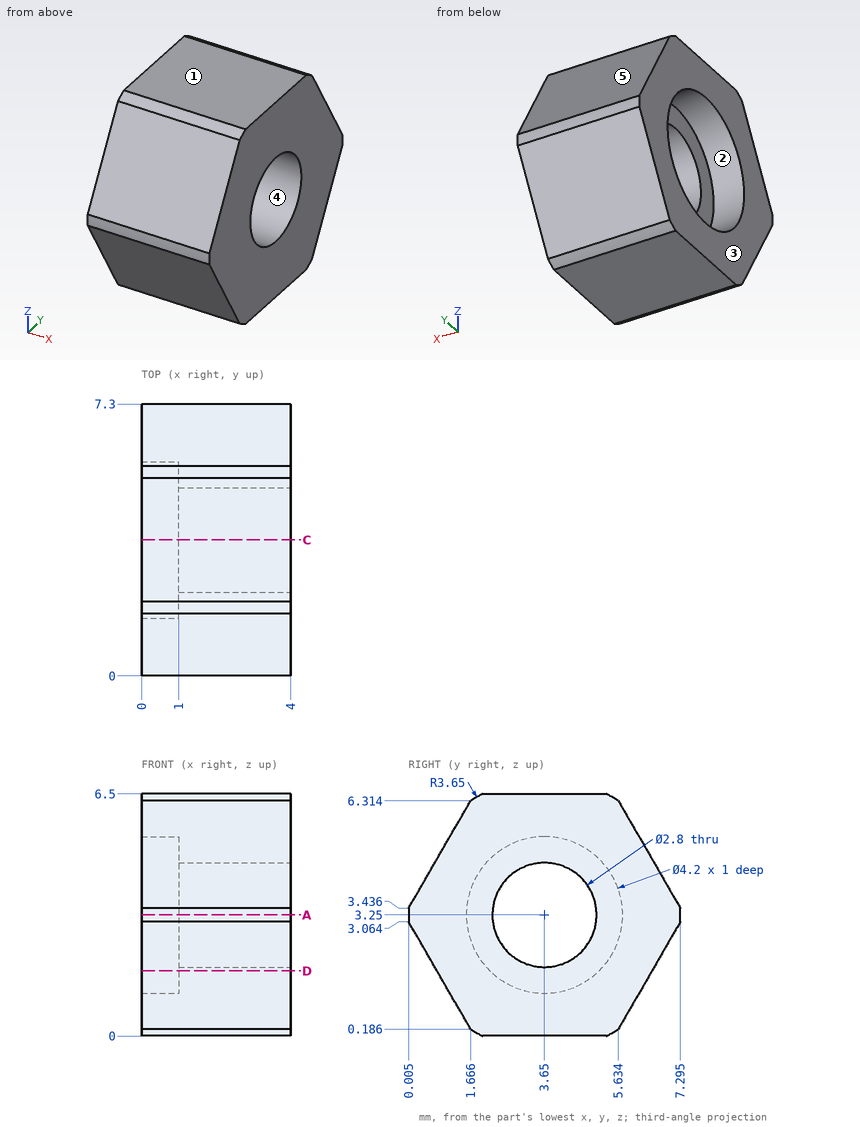
Geometry: see drawing. Coordinates: mm, zero at the bounding-box minimum. A direction names the side the tool comes from. Coordinates: 2 decimals unless noted, no trailing zeros. Order: outer loops, then holes, each group sorted by start corner. A loop starts at its lowest first (then second) coordinate and runs counter-clockwise, first axis right, second up. Notation, with made-up numbers: (-17, 38.25) -> (-5, 38.25) arc R26 cw to (-5, 64.25) -> close; hole circle Ø11 at (-2, 29). An arc over 180 degrees is marked (long way). Write each question's results on one line, items separated by ' | '. Start each with the question number.
1) Cut plane D-D, the plane z = 1.75. Output: boundary loops of the cut face in (x, y).
2) First-contact query: pin 1 (1.5 mm diameter, centred on x = 3, z = 0.5, fed in from -Y). Flat tip, straight axial feed; report the tip coordinate or a pass-through.
3) Cut plane C-C, the plane y = 3.65. Output: boundary loops of the cut face in (x, z), and give its area (3 significant figures).
4) Set-up query: the marked faces 1 and 2. Return all of +Z, -Z, +X, -X, +Y, -Y with unobstructed straight access to the full face (end or side cutting, diameter ignored); none if empty.
5) Cut plane A-A, the plane z = 3.25. Output: boundary loops of the cut face in (x, y), and give its area (3 significant figures).
6) Material intervals for line 1 along Z through (x, y) = (2.05, 3.65); line 2 along Y through (x, z) = (3.3, 2.5); line 3 along X through (y, z) = (3.5, 1.25), sorted ascending.
7) Mould query, pull axis Y, two halves, no side actions, for the marked faces 3, 4 and 5. Classes: released by +Y, released by -Y, zero draft, split by the parting line, or undercut.
Checks:
1) outline: (0, 0.76) -> (4, 0.76) -> (4, 6.54) -> (0, 6.54) -> (0, 5.12) -> (1, 5.12) -> (1, 2.18) -> (0, 2.18) -> close
2) pin 1: y = 1.05
3) outline: (0, 0) -> (4, 0) -> (4, 1.85) -> (1, 1.85) -> (1, 1.15) -> (0, 1.15) -> close; (0, 5.35) -> (1, 5.35) -> (1, 4.65) -> (4, 4.65) -> (4, 6.5) -> (0, 6.5) -> close | area: 13.4 mm^2
4) face 1: +Z, +X, -X, +Y, -Y | face 2: -X
5) outline: (0, 0) -> (4, 0) -> (4, 2.25) -> (1, 2.25) -> (1, 1.55) -> (0, 1.55) -> close; (0, 5.75) -> (1, 5.75) -> (1, 5.05) -> (4, 5.05) -> (4, 7.3) -> (0, 7.3) -> close | area: 16.6 mm^2
6) line 1: 0 to 1.85, 4.65 to 6.5 | line 2: 0.33 to 2.47, 4.83 to 6.97 | line 3: 1 to 4
7) face 3: zero draft | face 4: undercut | face 5: released by +Y
